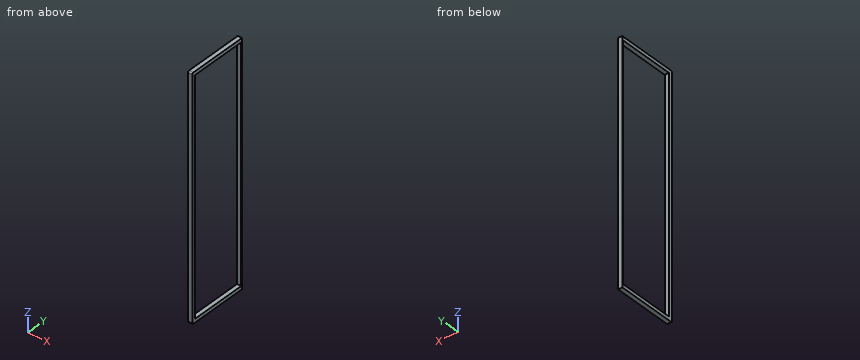
from build123d import *

# Parameters (mm, degrees)
SKETCH1_W           = 2000
SKETCH1_H           = 500
BOSS_EXTRUDE1_DEPTH = 35
SKETCH2_W           = 1940
SKETCH2_H           = 462.5
CUT_EXTRUDE1_DEPTH  = 35
FILLET1_R           = 10


with BuildPart() as part:
    # Sketch1 → Boss-Extrude1 (new body)
    with BuildSketch(Plane(origin=(0, 0, 0), x_dir=(0, 0, -1), z_dir=(1, 0, 0))):
        with Locations((-700.985902425, -1163.463280399)):
            Rectangle(SKETCH1_W, SKETCH1_H)
    extrude(amount=BOSS_EXTRUDE1_DEPTH)

    # Sketch2 → Cut-Extrude1 (cut)
    with BuildSketch(Plane(origin=(35, 0, 0), x_dir=(0, 0, -1), z_dir=(1, 0, 0))):
        with Locations((-700.985902425, -1152.213280399)):
            Rectangle(SKETCH2_W, SKETCH2_H)
    extrude(amount=-CUT_EXTRUDE1_DEPTH, mode=Mode.SUBTRACT)

    # Fillet1
    fillet1_edges = [part.edges().sort_by_distance(p)[0] for p in [
        (17.5, -1413.463280399, -299.014097575),
        (17.5, -1413.463280399, 1700.985902425),
    ]]
    fillet(fillet1_edges, radius=FILLET1_R)


solid = part.part
Work out the finished part from the listing and answer in its coordinate system (mm). Give positions to 0.01 mm unless a question says otherwise; leave off trailing zeros. Loops run counter-clockwise (first coordinate to the right, second up) from the corner with the lowest first, then second, coordinate; pieces in that order, holes last. Notation, with made-up numbers: (-15, 65) - (14, 65) arc R16 ccw to (14, 75) - close; hole circle Ø4 at (-33.5, 44.25). An arc over 180 degrees is marked (long way). Answer in a Markdown table with one row per item. Add a question column.
Q1. Consider line 1 along Z through (x, y) = (27.5, -1004); line 2 along Y through (x, z) = (22, 1326.5). Determine where each line is inside the solid, lowest interval first.
Q2. The part is cut by section C-C (x = 17). Determine the outline of the cut face in (y, z).
Q3. The part is cut by section A-A (z = 427.5). Determine the outline of the cut face in (x, y).
Q4. The part is cut by section B-B (y = -1163.5). Determine the outline of the cut face in (x, z), and give its area (3 significant figures).
Solution:
| question | item | result |
|---|---|---|
| 1 | line 1 | z = -299.01 to -269.01, 1670.99 to 1700.99 |
| 1 | line 2 | y = -1413.46 to -1383.46, -920.96 to -913.46 |
| 2 | outline | (-1413.46, -289.01) arc R10 ccw to (-1403.46, -299.01) - (-913.46, -299.01) - (-913.46, 1700.99) - (-1403.46, 1700.99) arc R10 ccw to (-1413.46, 1690.99) - close; hole (-1383.46, -269.01) - (-920.96, -269.01) - (-920.96, 1670.99) - (-1383.46, 1670.99) - close |
| 3 | outline | (0, -1413.46) - (35, -1413.46) - (35, -1383.46) - (0, -1383.46) - close; (0, -920.96) - (35, -920.96) - (35, -913.46) - (0, -913.46) - close |
| 4 | outline | (0, -299.01) - (35, -299.01) - (35, -269.01) - (0, -269.01) - close; (0, 1670.99) - (35, 1670.99) - (35, 1700.99) - (0, 1700.99) - close |
| 4 | area | 2,100 mm² |
